Design review of the part built by this model. Coordinates are the model's own, in mm. A direction names the side the tool comes from. Give positions to 0.01 mm unless a question says otherwise; leave off trailing zeros. Loops run counter-clockwise (first coordinate to the right, second up) from the corner with the lowest first, then second, coordinate; pieces in that order, holes last. Notation, with made-up numbers: M 79.25,-39.5 L 108.25,-39.5 A30 cw 108.25,-11.5 Z; hole C 4.5,24.5 d9. An arc over 180 degrees is marked long. Use CSV: the item, a comma, the result in double quotes.
from build123d import *

# Parameters (mm, degrees)
F0_R     = 15.621
F1_DEPTH = 11.43
F2_R     = 10.541
F3_DEPTH = 6.35
F4_R     = 17.78
F5_DEPTH = 2.54
F6_R     = 6.6675
F7_DEPTH = 17.781


with BuildPart() as f1:
    # F0 (on Top) → F1 (new body)
    with BuildSketch(Plane.XY):
        Circle(F0_R)
    extrude(amount=F1_DEPTH)

    # F2 (on face) → F3 (join)
    with BuildSketch(Plane.XY.offset(11.43)):
        Circle(F2_R)
    extrude(amount=F3_DEPTH)

    # F4 (on face) → F5 (join)
    with BuildSketch(Plane(origin=(0, 0, 0), x_dir=(1, 0, 0), z_dir=(0, 0, -1))):
        Circle(F4_R)
    extrude(amount=-F5_DEPTH)

    # F6 (on face) → F7 (cut, through all)
    with BuildSketch(Plane.XY.offset(17.78)):
        Circle(F6_R)
    extrude(amount=-F7_DEPTH, mode=Mode.SUBTRACT)

    # F8 (on Front) → F9 (revolve, cut)
    with BuildSketch(Plane.XZ):
        with BuildLine():
            ThreePointArc((9.779, 12.7), (7.64031, 14.850041), (6.858, 17.78))
            Line((6.858, 17.78), (1.041292, 17.78))
            Line((1.041292, 17.78), (1.041292, -3.794143))
            Line((1.041292, -3.794143), (10.795, -3.794143))
            Line((10.795, -3.794143), (10.795, 8.128))
            ThreePointArc((10.795, 8.128), (10.526845, 9.263923), (9.779, 10.16))
            Line((9.779, 10.16), (9.779, 12.7))
        make_face()
    revolve(axis=Axis((0, 0, 0.73688), (0, 0, -1)), mode=Mode.SUBTRACT)


solid = f1.part
(1) We need section D-D on y = 14.5. State the section outline as (x, z) points, then the cut area to 3 significant figures.
A:
outline,"M -10.29,0 L 10.29,0 L 10.29,2.54 L 5.81,2.54 L 5.81,11.43 L -5.81,11.43 L -5.81,2.54 L -10.29,2.54 Z"
area,"156 mm²"
(2) We need section A-A on y = 0. State the section outline as (x, z) points (3 decimals).
A:
outline,"M -17.78,0 L -10.795,0 L -10.795,8.128 A2.54 cw -9.779,10.16 L -9.779,12.7 A5.878 ccw -6.858,17.78 L -10.541,17.78 L -10.541,11.43 L -15.621,11.43 L -15.621,2.54 L -17.78,2.54 Z; M 6.858,17.78 A5.878 ccw 9.779,12.7 L 9.779,10.16 A2.54 cw 10.795,8.128 L 10.795,0 L 17.78,0 L 17.78,2.54 L 15.621,2.54 L 15.621,11.43 L 10.541,11.43 L 10.541,17.78 Z"
(3) Machinability: for faces 5 (the cylindrical face through (10.054, 3.166, 14.561)), 6 (the flat face through (8, 8, 0)), which of the approach directions +Z, -Z, +X, -X, +Y, -Y give a long, thin tool a straight path to every point of the face, cutting with its end or side? Answer none if there is none.
A:
face 5,"+Z"
face 6,"-Z, +X, -X, +Y, -Y"
(4) The part is to be moulded in two halves that separate along Y. For faces 1 (the cylindrical face through (-2.03, 15.49, 6.92)), 2 (the cylindrical face through (-7.956, -7.296, 4.121)), 3 (the cylindrical face through (-2.12, 9.546, 11.448)), 4 (the flat face through (10.2, -3.3, 11.43)), say which applies: released by +Y, released by -Y, zero draft, split by the parting line, or undercut.
A:
face 1,"split by the parting line"
face 2,"undercut"
face 3,"undercut"
face 4,"zero draft"
(5) Wall thickness on line 1 along Y through (x, z) = (0, 3.5) (3 decimals); line 2 along Y through (x, z) = (0, 2) (3 decimals): over which ranges is each line inside the solid? List them lowest first. Write a range as [from, to].
A:
line 1,"[-15.621, -10.795], [10.795, 15.621]"
line 2,"[-17.78, -10.795], [10.795, 17.78]"
(6) We need section B-B on z = 5.75. State the section outline as (x, y) points (3 decimals).
A:
outline,"C 0,0 d31.242; hole C 0,0 d21.59"
(7) Clearance check with flat-ended pins moving along their axes: P1, Ø2, axis at x = 1.5, z = 15.5, coming from the -Y side; P2, Ø3, axis at x = 13.5, y = 11.5, coming from the +Z side; P3, Ø10, axis at x = -8, z = 13.5, coming from the -Y side. State where each tip first meets the part, or that it passes through.
A:
P1,"y = -10.53"
P2,"z = 2.54"
P3,"y = -15.24"
